Geometry check sheet. Reference: drawing and pictorial views, mm from the part's lowest x, y, z. Give positions to 0.01 mm unless a question says otherwise; leave off trailing zeros. Write each loop counter-clockwise with the first axis right and the second up, starting at its lowest first coordinate (ties: lowest second). Pieces come first, ordered by that corner, then holes. Notation, with made-up numbers: (50.5, 62) -> (93.5, 62) arc R33 ccw to (93.5, 92) -> close; hole circle Ø10 at (-32.5, 39.5). An arc over 180 degrees is marked (long way). Use a Markdown table: item, result. Add a question column.
1. Cross-section at C-C (z = 50). Enter the section's corners in (x, y), then the cut area to 3 significant figures.
2. Cross-section at D-D (x = 26.5). Enter the section's corners in (y, z), then the cut area to 3 significant figures.
3. Cross-section at A-A (z = 35). Enter the section's corners in (x, y), then the cut area to 3 significant figures.
4. Gauge pin test, flat ends, axial feed: P1, Ø10, axis at x = 9.02, z = 50, coming from the -Y side; P2, Ø2, axis at x = 62, z = 49.5, coming from the -Y side; P3, Ø3, axis at y = 3, z = 34.5, coming from the +X side. Record the tip position at first contact, or that the pin passes through.
5. Release check for a two-part mould opening along X. For the marked faces 1, 2 and 3 record: released by +X, released by -X, zero draft, split by the parting line, or undercut.
6. Scan lines: probe 1 along X at (y, z) = (1.25, 50); probe 2 along X at (y, z) = (3.95, 20); probe 3 along Z at (x, y) = (60, 2.2) (1 decimal). Record each from-to range of solid material in increasing order. Write a range as [from, to].
7. Cross-section at B-B (x = 35). Enter the section's corners in (y, z), then the cut area to 4 significant figures.
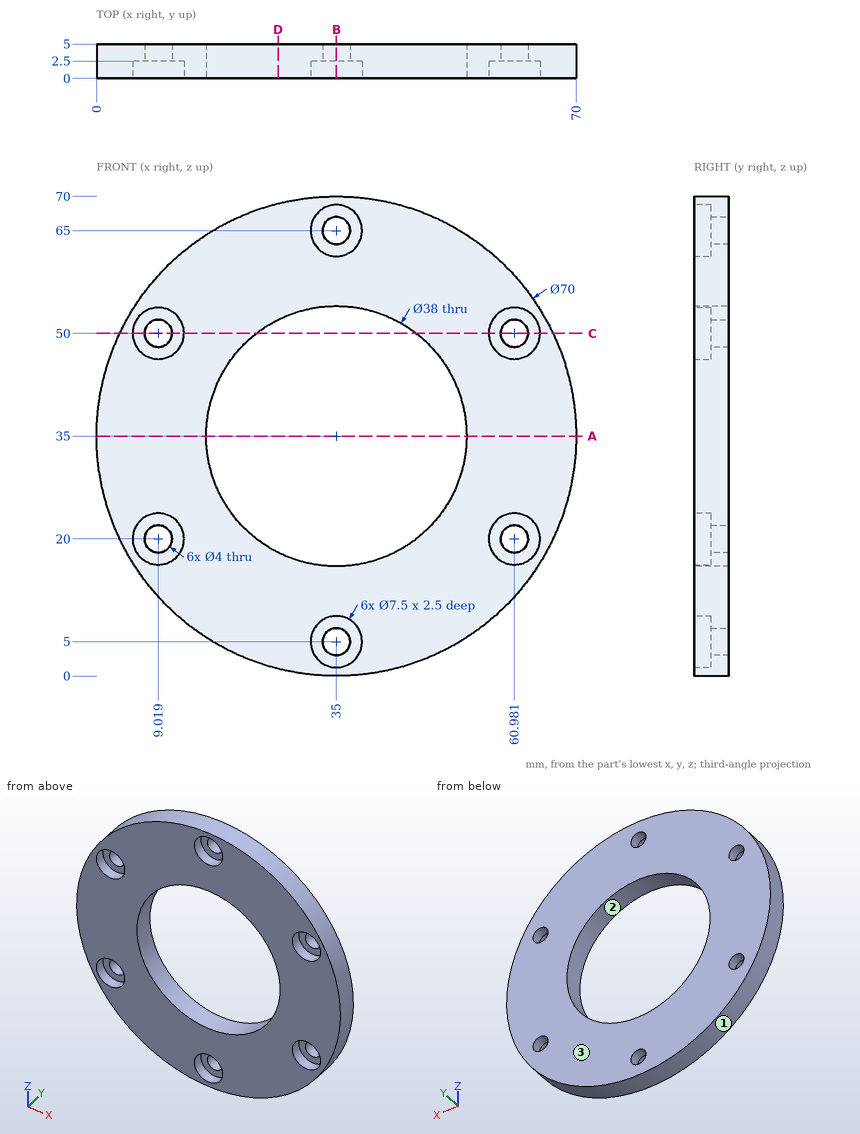
Worked answers:
| question | item | result |
|---|---|---|
| 1 | outline | (3.38, 0) -> (5.27, 0) -> (5.27, 2.5) -> (7.02, 2.5) -> (7.02, 5) -> (3.38, 5) -> close; (11.02, 2.5) -> (12.77, 2.5) -> (12.77, 0) -> (23.34, 0) -> (23.34, 5) -> (11.02, 5) -> close; (46.66, 0) -> (57.23, 0) -> (57.23, 2.5) -> (58.98, 2.5) -> (58.98, 5) -> (46.66, 5) -> close; (62.98, 2.5) -> (64.73, 2.5) -> (64.73, 0) -> (66.62, 0) -> (66.62, 5) -> (62.98, 5) -> close |
| 1 | area | 142 mm² |
| 2 | outline | (0, 1.05) -> (5, 1.05) -> (5, 18.01) -> (0, 18.01) -> close; (0, 51.99) -> (5, 51.99) -> (5, 68.95) -> (0, 68.95) -> close |
| 2 | area | 170 mm² |
| 3 | outline | (0, 0) -> (16, 0) -> (16, 5) -> (0, 5) -> close; (54, 0) -> (70, 0) -> (70, 5) -> (54, 5) -> close |
| 3 | area | 160 mm² |
| 4 | P1 | stops at y = 0 |
| 4 | P2 | stops at y = 2.5 |
| 4 | P3 | stops at x = 70 |
| 5 | face 1 | split by the parting line |
| 5 | face 2 | undercut |
| 5 | face 3 | zero draft |
| 6 | probe 1 | x = [3.38, 5.27], [12.77, 23.34], [46.66, 57.23], [64.73, 66.62] |
| 6 | probe 2 | x = [3.38, 7.02], [11.02, 23.34], [46.66, 58.98], [62.98, 66.62] |
| 6 | probe 3 | z = [10.5, 16.4], [23.6, 46.4], [53.6, 59.5] |
| 7 | outline | (0, 0) -> (5, 0) -> (5, 3) -> (2.5, 3) -> (2.5, 1.25) -> (0, 1.25) -> close; (0, 8.75) -> (2.5, 8.75) -> (2.5, 7) -> (5, 7) -> (5, 16) -> (0, 16) -> close; (0, 54) -> (5, 54) -> (5, 63) -> (2.5, 63) -> (2.5, 61.25) -> (0, 61.25) -> close; (0, 68.75) -> (2.5, 68.75) -> (2.5, 67) -> (5, 67) -> (5, 70) -> (0, 70) -> close |
| 7 | area | 102.5 mm² |
